Verification items for the finished model (mm, model axes). A direction names the side the tool comes from. Round coordinates to 2 decimals unless told otherwise and drop trailing zeros. Answer as a JSON object with one key per item and string values.
```python
from build123d import *

# Parameters (mm, degrees)
F1_R      = 2.6
F2_DEPTH  = 12
F3_W      = 43.75
F3_H      = 43.75
F4_DEPTH  = 6
F5_R      = 2.5
F6_R      = 2.1
F7_DEPTH  = 25
F10_DEPTH = 1.5
F8_R      = 4
F11_DEPTH = 1.5
F12_R     = 2.1
F13_DEPTH = 25
F14_SIZE  = 1


with BuildPart() as f2:
    # F1 (on Top) → F2 (new body)
    with BuildSketch(Plane.XY):
        with BuildLine():
            Line((-57.5, -72.5), (57.5, -72.5))
            ThreePointArc((57.5, -72.5), (61.035534, -71.035534), (62.5, -67.5))
            Line((62.5, -67.5), (62.5, 67.5))
            ThreePointArc((62.5, 67.5), (61.035534, 71.035534), (57.5, 72.5))
            Line((57.5, 72.5), (-57.5, 72.5))
            ThreePointArc((-57.5, 72.5), (-61.035534, 71.035534), (-62.5, 67.5))
            Line((-62.5, 67.5), (-62.5, -67.5))
            ThreePointArc((-62.5, -67.5), (-61.035534, -71.035534), (-57.5, -72.5))
        make_face()
        with Locations((-30, -67.5)):
            Circle(F1_R, mode=Mode.SUBTRACT)
        with Locations((30, -67.5)):
            Circle(F1_R, mode=Mode.SUBTRACT)
        with Locations((-30, 67.5)):
            Circle(F1_R, mode=Mode.SUBTRACT)
        with Locations((30, 67.5)):
            Circle(F1_R, mode=Mode.SUBTRACT)
    extrude(amount=F2_DEPTH)

    # F3 (on face) → F4 (cut)
    with BuildSketch(Plane.XY.offset(12)):
        with BuildLine():
            Line((-50, -55), (50, -55))
            ThreePointArc((50, -55), (53.535534, -53.535534), (55, -50))
            Line((55, -50), (55, 50))
            ThreePointArc((55, 50), (53.535534, 53.535534), (50, 55))
            Line((50, 55), (-50, 55))
            ThreePointArc((-50, 55), (-53.535534, 53.535534), (-55, 50))
            Line((-55, 50), (-55, -50))
            ThreePointArc((-55, -50), (-53.535534, -53.535534), (-50, -55))
        make_face()
        with Locations((-25.625, -25.625)):
            Rectangle(F3_W, F3_H, mode=Mode.SUBTRACT)
        with Locations((25.625, -25.625)):
            Rectangle(F3_W, F3_H, mode=Mode.SUBTRACT)
        with Locations((-25.625, 25.625)):
            Rectangle(F3_W, F3_H, mode=Mode.SUBTRACT)
        with Locations((25.625, 25.625)):
            Rectangle(F3_W, F3_H, mode=Mode.SUBTRACT)
    extrude(amount=-F4_DEPTH, mode=Mode.SUBTRACT)

    # F5
    f5_edges = [f2.edges().sort_by_distance(p)[0] for p in [
        (0, -55, 6),
        (53.535534, -53.535534, 6),
        (55, 0, 6),
        (53.535534, 53.535534, 6),
        (0, 55, 6),
        (-53.535534, 53.535534, 6),
        (-55, 0, 6),
        (-53.535534, -53.535534, 6),
        (-25.625, -47.5, 6),
        (-47.5, -25.625, 6),
        (-25.625, -3.75, 6),
        (-3.75, -25.625, 6),
        (47.5, -25.625, 6),
        (25.625, -47.5, 6),
        (3.75, -25.625, 6),
        (25.625, -3.75, 6),
        (-25.625, 3.75, 6),
        (-47.5, 25.625, 6),
        (-25.625, 47.5, 6),
        (-3.75, 25.625, 6),
        (25.625, 47.5, 6),
        (47.5, 25.625, 6),
        (25.625, 3.75, 6),
        (3.75, 25.625, 6),
    ]]
    fillet(f5_edges, radius=F5_R)

    # F6 (on face) → F7 (cut)
    with BuildSketch(Plane.XY.offset(12)):
        with Locations((-25.625, 25.625)):
            Circle(F6_R)
        with Locations((25.625, 25.625)):
            Circle(F6_R)
        with Locations((25.625, -25.625)):
            Circle(F6_R)
        with Locations((-25.625, -25.625)):
            Circle(F6_R)
    extrude(amount=-F7_DEPTH, mode=Mode.SUBTRACT)

    # F9 (on face) → F10 (cut)
    with BuildSketch(Plane.XY.offset(12)):
        with BuildLine():
            Line((50, 59), (-50, 59))
            ThreePointArc((-50, 59), (-56.363961, 56.363961), (-59, 50))
            Line((-59, 50), (-59, -50))
            ThreePointArc((-59, -50), (-56.363961, -56.363961), (-50, -59))
            Line((-50, -59), (50, -59))
            ThreePointArc((50, -59), (56.363961, -56.363961), (59, -50))
            Line((59, -50), (59, 50))
            ThreePointArc((59, 50), (56.363961, 56.363961), (50, 59))
        make_face()
        with BuildLine():
            ThreePointArc((57, -50), (54.949747, -54.949747), (50, -57))
            Line((50, -57), (-50, -57))
            ThreePointArc((-50, -57), (-54.949747, -54.949747), (-57, -50))
            Line((-57, -50), (-57, 50))
            ThreePointArc((-57, 50), (-54.949747, 54.949747), (-50, 57))
            Line((-50, 57), (50, 57))
            ThreePointArc((50, 57), (54.949747, 54.949747), (57, 50))
            Line((57, 50), (57, -50))
        make_face(mode=Mode.SUBTRACT)
    extrude(amount=-F10_DEPTH, mode=Mode.SUBTRACT)

    # F8 (on face) → F11 (cut)
    with BuildSketch(Plane.XY.offset(12)):
        with Locations((-25.625, 25.625)):
            Circle(F8_R)
        with Locations((-25.625, -25.625)):
            Circle(F8_R)
        with Locations((25.625, 25.625)):
            Circle(F8_R)
        with Locations((25.625, -25.625)):
            Circle(F8_R)
    extrude(amount=-F11_DEPTH, mode=Mode.SUBTRACT)

    # F12 (on face) → F13 (cut)
    with BuildSketch(Plane.XZ.offset(72.5)):
        with Locations((0, 5)):
            Circle(F12_R)
    extrude(amount=-F13_DEPTH, mode=Mode.SUBTRACT)

    # F14
    f14_edges = [f2.edges().sort_by_distance(p)[0] for p in [
        (-0.551164, -47.5, 2.97362),
    ]]
    chamfer(f14_edges, length=F14_SIZE)


solid = f2.part
```
1. Go/stop test with flat-tipped pins: pin 1 (1.7 mm diameter, centred on x = 0, z = 4.5, fed in from -Y); pin 2 (9 mm diameter, centred on x = -25.625, y = 25.625, fed in from +Z); pin 3 (2.5 mm diameter, centred on x = -24.5, y = 27.5, fed in from +Z). Record where each tip stops, or that it passes through.
Completed:
{"pin 1": "stops at y = -47.75", "pin 2": "stops at z = 12", "pin 3": "stops at z = 10.5"}
2. Material ranges on probe 1 along Y at (x, z) = (-14.5, 9); probe 2 along Y at (x, z) = (30, 9); probe 3 along Y at (x, z) = (-36, 6.75), recorded low to high. Write a range as from..to.
Completed:
{"probe 1": "y = -72.5..-55, -47.5..-3.75, 3.75..47.5, 55..72.5", "probe 2": "y = -72.5..-70.1, -64.9..-55, -47.5..-3.75, 3.75..47.5, 55..64.9, 70.1..72.5", "probe 3": "y = -72.5..-54.29, -48.21..-3.04, 3.04..48.21, 54.29..72.5"}
3. Mould release check, pull along X, two halves, no side actions. Record for faces 3 (the face through (30, 26, 12)), 4 (the face through (-62.5, 1, 6)), 5 (the face through (0, -4, 6)): released by +X, released by -X, zero draft, split by the parting line, or undercut.
Completed:
{"face 3": "zero draft", "face 4": "released by -X", "face 5": "undercut"}
4. Access from +Z, -Z, +X, -X, +Y, -Y to the whole of each face (thin tool, end or side, straight path). Record for faces 1 (the face through (-53, 54, 10)), 2 (the face through (-1, 1, 0)).
Completed:
{"face 1": "+Z", "face 2": "-Z, +X, -X, +Y, -Y"}
